```python
from build123d import *

# Parameters (mm, degrees)
SKETCH_1_R          = 1.55
EXTRUDE_1_DEPTH     = 10
CUT_EXTRUDE_1_REACH = 46.159
SKETCH_3_R          = 1.55
CUT_EXTRUDE_2_REACH = 46.159
SKETCH_4_R          = 1.55


with BuildPart() as part:
    # 草图1 → 凸台-拉伸1 (new body)
    with BuildSketch(Plane(origin=(0, 0, 0), x_dir=(1, 0, 0), z_dir=(0, 1, 0))):
        Polygon((0, 0), (25, 0), (25, -10), (10, -10), (10, -25), (25, -25), (25, -35), (0, -35), align=None)
        with Locations(Location((5, -17.5, 0), (0, 0, 270))):
            Circle(SKETCH_1_R, mode=Mode.SUBTRACT)
        with Locations(Location((17.5, -5, 0), (0, 0, 270))):
            Circle(SKETCH_1_R, mode=Mode.SUBTRACT)
        with Locations(Location((17.5, -30, 0), (0, 0, 270))):
            Circle(SKETCH_1_R, mode=Mode.SUBTRACT)
    extrude(amount=EXTRUDE_1_DEPTH)

    # 切除-拉伸1: up to this face of the body (flat: up to its plane)
    cut_extrude_1_end = Plane(part.part.faces().sort_by_distance((10, 5, 17.5))[0])
    # 草图3 → 切除-拉伸1 (cut, up to the picked face)
    with BuildSketch(Plane.ZY, mode=Mode.PRIVATE) as cut_extrude_1_sk1:
        with Locations((17.5, 5)):
            Circle(SKETCH_3_R)
    cut_extrude_1_tool1 = split(extrude(cut_extrude_1_sk1.sketch, amount=-CUT_EXTRUDE_1_REACH, mode=Mode.PRIVATE), bisect_by=cut_extrude_1_end, keep=Keep.BOTH, mode=Mode.PRIVATE)
    add(cut_extrude_1_tool1.solids().sort_by(Axis((0, 5, 17.5), (1, 0, 0)))[0], mode=Mode.SUBTRACT)

    # 切除-拉伸2: up to this face of the body (flat: up to its plane)
    cut_extrude_2_end = Plane(part.part.faces().sort_by_distance((12.5, 5, 0))[0])
    # 草图4 → 切除-拉伸2 (cut, up to the picked face)
    with BuildSketch(Plane.XY.offset(35), mode=Mode.PRIVATE) as cut_extrude_2_sk1:
        with Locations((17.5, 5)):
            Circle(SKETCH_4_R)
    cut_extrude_2_tool1 = split(extrude(cut_extrude_2_sk1.sketch, amount=-CUT_EXTRUDE_2_REACH, mode=Mode.PRIVATE), bisect_by=cut_extrude_2_end, keep=Keep.BOTH, mode=Mode.PRIVATE)
    add(cut_extrude_2_tool1.solids().sort_by(Axis((17.5, 5, 35), (0, 0, -1)))[0], mode=Mode.SUBTRACT)


solid = part.part
```
Input: part model. Units: mm. Frame: model coordinates. A direction names the side the tool comes from. Coordinates: 2 decimals unless noted, no trailing zeros. Loops run counter-clockwise (first coordinate to the right, second up) from the corner with the lowest first, then second, coordinate; pieces in that order, holes last. Notation, with made-up numbers: M -8.75,34 L 48.25,34 A20 cw 48.25,62 Z; hole C 52,37.5 d11. An arc over 180 degrees is marked long. One line per item, written item: value.
(1) Line query: line 1 along Z through (x, y) = (13.75, 5.75); line 2 along X through (y, z) = (5, 28.2); line 3 along X through (y, z) = (8.45, 17.5). Output: solid intervals per line, ascending. Write a range as from..to.
Filled in:
line 1: 0..10, 25..35
line 2: 0..15.95, 19.05..25
line 3: 0..3.45, 6.55..10
(2) Section A-A (x = 13.5). Output: boundary loops of the cut face in (y, z).
Filled in:
outline: M 0,0 L 10,0 L 10,10 L 0,10 Z; M 0,25 L 10,25 L 10,35 L 0,35 Z
(3) Section C-C (y = 6). Give the number of separate pieces and of enclosed holes in the cut face, and give its area (3 significant figures).
Filled in:
separate pieces: 4
enclosed holes: 0
area: 576 mm^2
(4) Reachability of faces 1 (the cylindrical face through (6.537, 8.021, 17.298)), 2 (the flat face through (19.3, 4.9, 10)) from +Z, -Z, +X, -X, +Y, -Y: full face, straight path, thin tool, end or side. Return the list, or none.
Filled in:
face 1: +Y, -Y
face 2: +X, +Y, -Y
(5) Pull-direction query (Y, two-part tool) for faces 3 (the cylindrical face through (17.298, 6.537, 1.979)), 4 (the flat face through (7, 0, 17)), 5 (the cylindrical face through (5.466, 1.909, 18.978)); classes: +Y half, -Y half, draft (parallel to the pull), parting line (faces both ways), or undercut.
Filled in:
face 3: undercut
face 4: -Y half
face 5: draft
(6) Pin query (flat end, axial travel): pin 1 (3 mm diameter, centred on y = 9, z = 13.5, fed in from +X); pin 2 (3 mm diameter, centred on x = 17.5, y = 5, fed in from -Z). Return the tip coordinate at first contact, or that it passes through.
Filled in:
pin 1: x = 10
pin 2: through
(7) Section B-B (z = 17.5). Output: boundary loops of the cut face in (x, y), and give its area (3 significant figures).
Filled in:
outline: M 0,0 L 3.45,0 L 3.45,3.45 L 0,3.45 Z; M 0,6.55 L 3.45,6.55 L 3.45,10 L 0,10 Z; M 6.55,0 L 10,0 L 10,3.45 L 6.55,3.45 Z; M 6.55,6.55 L 10,6.55 L 10,10 L 6.55,10 Z
area: 47.6 mm^2
